```python
from build123d import *

# Parameters (mm, degrees)
SKETCH1_W           = 5
SKETCH1_H           = 105
BOSS_EXTRUDE1_DEPTH = 5
BOSS_EXTRUDE2_START = 129
BOSS_EXTRUDE2_DEPTH = 15
BOSS_EXTRUDE3_START = 129
SKETCH3_W           = 33.371379062
SKETCH3_H           = 5
BOSS_EXTRUDE3_DEPTH = 15
SKETCH4_W           = 3
SKETCH4_H           = 3.016632821
SKETCH4_H_2         = 3
BOSS_EXTRUDE4_DEPTH = 46
FILLET1_R           = 0.5
FILLET2_R           = 0.1
FILLET3_R           = 3
LPATTERN2_COUNT     = 2
LPATTERN2_PITCH     = 20
CUT_EXTRUDE3_DEPTH  = 29
CUT_EXTRUDE4_DEPTH  = 106


with BuildPart() as part:
    # Sketch1 → Boss-Extrude1 (new body)
    with BuildSketch(Plane(origin=(0, -9.496519724, 0), x_dir=(1, 0, 0), z_dir=(0, 1, 0))):
        with Locations((177.597354305, -136.516632821)):
            Rectangle(SKETCH1_W, SKETCH1_H)
    boss_extrude1 = extrude(amount=BOSS_EXTRUDE1_DEPTH)

    # Sketch2 → Boss-Extrude2 (add)
    with BuildSketch(Plane(origin=(0, -9.496519724, 0), x_dir=(1, 0, 0), z_dir=(0, 0, 1)).offset(BOSS_EXTRUDE2_START)):
        Polygon((180.097354305, 5), (175.549258031, 48.019997969), (175.549258031, 5), align=None)
    extrude(amount=BOSS_EXTRUDE2_DEPTH)

    # Sketch3 → Boss-Extrude3 (add)
    with BuildSketch(Plane(origin=(0, -9.496519724, 0), x_dir=(1, 0, 0), z_dir=(0, 0, 1)).offset(BOSS_EXTRUDE3_START)):
        with Locations((158.411664774, 2.5)):
            Rectangle(SKETCH3_W, SKETCH3_H)
    extrude(amount=BOSS_EXTRUDE3_DEPTH)

    # Sketch4 → Boss-Extrude4 (add)
    with BuildSketch(Plane(origin=(0, -9.496519724, 0), x_dir=(1, 0, 0), z_dir=(0, 1, 0))):
        with Locations((143.225975243, -145.508316411)):
            Rectangle(SKETCH4_W, SKETCH4_H)
        with Locations((143.225975243, -127.516632821)):
            Rectangle(SKETCH4_W, SKETCH4_H_2)
    extrude(amount=BOSS_EXTRUDE4_DEPTH)

    # Fillet1
    fillet1_edges = [part.edges().sort_by_distance(p)[0] for p in [
        (144.725975243, 36.503480276, 145.50831641),
        (143.225975243, 36.503480276, 144),
        (141.725975243, 36.503480276, 145.50831641),
        (143.225975243, 36.503480276, 147.016632821),
        (144.725975243, 36.503480276, 127.516632821),
        (143.225975243, 36.503480276, 126.016632821),
        (141.725975243, 36.503480276, 127.516632821),
        (143.225975243, 36.503480276, 129.016632821),
    ]]
    fillet(fillet1_edges, radius=FILLET1_R)

    # Fillet2
    fillet2_edges = [part.edges().sort_by_distance(p)[0] for p in [
        (175.549258031, 38.523478245, 136.5),
    ]]
    fillet(fillet2_edges, radius=FILLET2_R)

    # Fillet3
    fillet3_edges = [part.edges().sort_by_distance(p)[0] for p in [
        (177.823306168, -4.496519724, 129),
        (177.823306168, -4.496519724, 144),
    ]]
    fillet(fillet3_edges, radius=FILLET3_R)

    # LPattern2: Boss-Extrude1 ×2
    with Locations(*[(-i * LPATTERN2_PITCH, 0, 0) for i in range(1, LPATTERN2_COUNT)]):
        add(boss_extrude1)

    # Sketch7 → Cut-Extrude3 (cut)
    with BuildSketch(Plane(origin=(180.097354305, 0, 0), x_dir=(0, 0, -1), z_dir=(1, 0, 0))):
        Polygon((-129.016632821, -6.996519724), (-130.674945216, -9.496519724), (-84.016632821, -9.496519724), (-84.016632821, -6.996519724), align=None)
        Polygon((-189.016632821, -6.996519724), (-189.016632821, -9.496519724), (-142.358320426, -9.496519724), (-144.016632821, -6.996519724), align=None)
    extrude(amount=-CUT_EXTRUDE3_DEPTH, mode=Mode.SUBTRACT)

    # Sketch11 → Cut-Extrude4 (cut)
    with BuildSketch(Plane(origin=(0, 0, 84.016632821), x_dir=(-1, 0, 0), z_dir=(0, 0, -1))):
        Polygon((-178.097354305, -6.996519724), (-178.097354305, -5.996519724), (-179.097354305, -5.996519724), (-179.097354305, 4.208174), (-176.097354305, 4.208174), (-176.097354305, -5.996519724), (-177.097354305, -5.996519724), (-177.097354305, -6.996519724), align=None)
    extrude(amount=-CUT_EXTRUDE4_DEPTH, mode=Mode.SUBTRACT)


solid = part.part
```
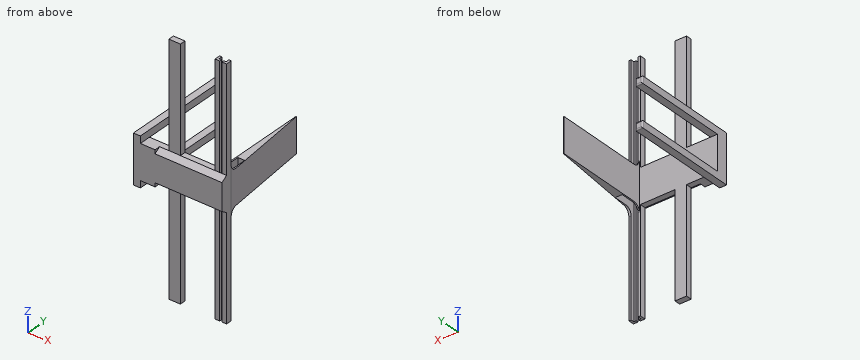
CAD build for the part. Positions are in the model's coordinates, mm. Round coordinates to 2 decimals unless told otherwise and drop trailing zeros. Order: outer loops, then holes, each group sorted by start corner. A loop starts at its lowest first (then second) coordinate and runs counter-clockwise, first axis right, second up.
Q1. Wall check: L1, parallel to Z at x = 144, y = 10; L2, parallel to Y at x = 160, z = 107.5; L3, parallel to Y at x = 161, z = 142.5. Give the ranges that are in metal, low to high.
Q2. Slice it at D-D (z = 180). Write the cut outline in (x, y), and give its area (3 significant figures).
Q3. Drop flat-ended pins along their axis: pin 1 (10 mm diameter, centred on x = 150, z = 129, fed in from +Y); pin 2 (3 mm diameter, centred on x = 176, y = 6, fed in from -Z); pin 3 (1 mm diameter, centred on y = 29.5, z = 137, fed in from -X). Give the stop position or say it passes through.
Q4. Slice it at A-A (z = 134.5). Write the cut outline in (x, y).
Q5. Slice it at B-B (y = 8). Write the cut outline in (x, z).
Results below:
1. L1: z = 126.02 to 129.02, 144 to 147.02
1. L2: y = -7 to -4.5
1. L3: y = -9.28 to -4.5
2. outline: (155.1, -7) - (160.1, -7) - (160.1, -4.5) - (155.1, -4.5) - close; (175.1, -7) - (177.1, -7) - (177.1, -6) - (176.1, -6) - (176.1, -4.5) - (175.1, -4.5) - close; (178.1, -7) - (180.1, -7) - (180.1, -4.5) - (179.1, -4.5) - (179.1, -6) - (178.1, -6) - close
2. area: 19.5 mm2
3. pin 1: stops at y = -4.5
3. pin 2: stops at z = 129
3. pin 3: stops at x = 175.55
4. outline: (141.73, -9.5) - (180.1, -9.5) - (180.1, -4.5) - (175.75, 36.64) arc R0.1 ccw to (175.55, 36.63) - (175.55, -4.5) - (141.73, -4.5) - close; hole (176.1, -6) - (177.1, -6) - (177.1, -7) - (178.1, -7) - (178.1, -6) - (179.1, -6) - (179.1, 4.21) - (176.1, 4.21) - close
5. outline: (141.73, 126.02) - (144.73, 126.02) - (144.73, 129.02) - (141.73, 129.02) - close; (141.73, 144) - (144.73, 144) - (144.73, 147.02) - (141.73, 147.02) - close; (175.55, 129) - (178.78, 129) - (178.78, 144) - (175.55, 144) - close
